Input: part model. Units: mm. Frame: model coordinates. Face numbers are marked on the shaded views. A direction names the side the tool comes from. Give positions to 0.01 mm unless a question says otherwise; leave off trailing zeros. Order: outer loops, then holes, each group sorted by start corner. A loop starts at its lowest first (then second) coordinate and runs counter-clockwise, first axis right, second up. Notation, with made-up numbers: (10.5, 46) - (55.5, 46) arc R19 cw to (55.5, 69) - close; hole circle Ø11 at (25.5, 89). An arc over 180 degrees is marked (long way). Answer in a Markdown table with one row per item. Add a question column.
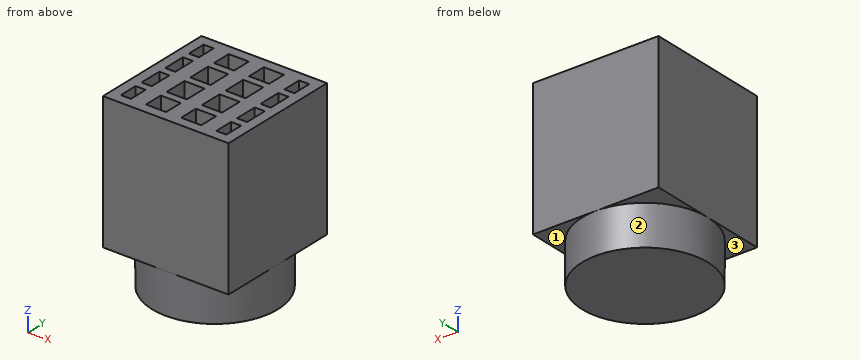
from build123d import *

# Parameters (mm, degrees)
SKETCH_8_W       = 25
SKETCH_8_H       = 25
SKETCH_8_W_2     = 4
SKETCH_8_H_2     = 21
SKETCH_8_W_3     = 2
EXTRUDE_7_DEPTH  = 25
SKETCH_9_W       = 25
SKETCH_9_H       = 25
EXTRUDE_8_DEPTH  = 2
SKETCH_14_W      = 25
SKETCH_14_H      = 1.5
EXTRUDE_11_DEPTH = 25
SKETCH_16_R      = 12.5
SKETCH_16_R_2    = 10
EXTRUDE_14_DEPTH = 6
SKETCH_17_R      = 12.5
EXTRUDE_15_DEPTH = 2


with BuildPart() as part:
    # 草图8 → 凸台-拉伸7 (new body)
    with BuildSketch(Plane.XY):
        Rectangle(SKETCH_8_W, SKETCH_8_H)
        with Locations((3.5, 0)):
            Rectangle(SKETCH_8_W_2, SKETCH_8_H_2, mode=Mode.SUBTRACT)
        with Locations((-3.5, 0)):
            Rectangle(SKETCH_8_W_2, SKETCH_8_H_2, mode=Mode.SUBTRACT)
        with Locations((-9.5, 0)):
            Rectangle(SKETCH_8_W_3, SKETCH_8_H_2, mode=Mode.SUBTRACT)
        with Locations((9.5, 0)):
            Rectangle(SKETCH_8_W_3, SKETCH_8_H_2, mode=Mode.SUBTRACT)
    extrude(amount=EXTRUDE_7_DEPTH)

    # 草图9 → 凸台-拉伸8 (add)
    with BuildSketch(Plane(origin=(0, 0, 0), x_dir=(-1, 0, 0), z_dir=(0, 0, -1))):
        Rectangle(SKETCH_9_W, SKETCH_9_H)
    extrude(amount=EXTRUDE_8_DEPTH)

    # 草图14 → 凸台-拉伸11 (add)
    with BuildSketch(Plane.XY.offset(25)):
        Rectangle(SKETCH_14_W, SKETCH_14_H)
        with Locations((0, 6)):
            Rectangle(SKETCH_14_W, SKETCH_14_H)
        with Locations((0, -6)):
            Rectangle(SKETCH_14_W, SKETCH_14_H)
    extrude(amount=-EXTRUDE_11_DEPTH)

    # 草图16 → 凸台-拉伸14 (add)
    with BuildSketch(Plane(origin=(0, 0, -2), x_dir=(-1, 0, 0), z_dir=(0, 0, -1))):
        Circle(SKETCH_16_R)
        Circle(SKETCH_16_R_2, mode=Mode.SUBTRACT)
    extrude(amount=EXTRUDE_14_DEPTH)

    # 草图17 → 凸台-拉伸15 (add)
    with BuildSketch(Plane(origin=(0, 0, -8), x_dir=(-1, 0, 0), z_dir=(0, 0, -1))):
        Circle(SKETCH_17_R)
    extrude(amount=EXTRUDE_15_DEPTH)


solid = part.part
Q1. Section A-A, the plane y = -6. Return loops of the section in (x, z), then the cut area to 3 significant figures.
Q2. Section B-B, the plane z = 15.5. State how many separate pieces and enclosed holes the cut face has, then the cut area to 3 significant figures.
Q3. Contact query for a flat-ended pin moving along its axis: P1, Ø1.2, axis at x = -2.5, y = -2.5, coming from the +Z side. Output: stop coordinate, or through.
Q4. Line query: probe 1 along X at (y, z) = (1.5, 19); probe 2 along Z at (x, y) = (-5, -2.25); probe 3 along Y at (x, z) = (0, -4.3). Output: solid intervals per line, ascending.
Q5. Section C-C, the plane x = 1. Return loops of the section in (y, z), then the cut area to 3 significant figures.
Q6. Section D-D, the plane x = -5. Return loops of the section in (y, z), then the cut area to 3 significant figures.
Q7. Access query for the marked faces 1, 2 and 3. Directions: +Z, -Z, +X, -X, +Y, -Y. A direction counts if a zero-diameter tool reaches every point of the face in a straight line with its end or side. Return the directions, or none.
Computed:
| question | item | result |
|---|---|---|
| 1 | outline | (-12.5, -2) - (-10.97, -2) - (-10.97, -10) - (10.97, -10) - (10.97, -2) - (12.5, -2) - (12.5, 25) - (-12.5, 25) - close; hole (-8, -8) - (8, -8) - (8, -2) - (-8, -2) - close |
| 1 | area | 754 mm^2 |
| 2 | separate pieces | 1 |
| 2 | enclosed holes | 16 |
| 2 | area | 427 mm^2 |
| 3 | P1 | stops at z = 0 |
| 4 | probe 1 | x = -12.5 to -10.5, -8.5 to -5.5, -1.5 to 1.5, 5.5 to 8.5, 10.5 to 12.5 |
| 4 | probe 2 | z = -10 to -8, -2 to 0 |
| 4 | probe 3 | y = -12.5 to -10, 10 to 12.5 |
| 5 | outline | (-12.5, -2) - (-12.46, -2) - (-12.46, -10) - (12.46, -10) - (12.46, -2) - (12.5, -2) - (12.5, 25) - (-12.5, 25) - close; hole (-9.95, -8) - (9.95, -8) - (9.95, -2) - (-9.95, -2) - close |
| 5 | area | 755 mm^2 |
| 6 | outline | (-12.5, -2) - (-11.46, -2) - (-11.46, -10) - (11.46, -10) - (11.46, -2) - (12.5, -2) - (12.5, 25) - (10.5, 25) - (10.5, 0) - (6.75, 0) - (6.75, 25) - (5.25, 25) - (5.25, 0) - (0.75, 0) - (0.75, 25) - (-0.75, 25) - (-0.75, 0) - (-5.25, 0) - (-5.25, 25) - (-6.75, 25) - (-6.75, 0) - (-10.5, 0) - (-10.5, 25) - (-12.5, 25) - close; hole (-8.66, -8) - (8.66, -8) - (8.66, -2) - (-8.66, -2) - close |
| 6 | area | 342 mm^2 |
| 7 | face 1 | -Z, +X, +Y |
| 7 | face 2 | -Z |
| 7 | face 3 | -Z, -X, -Y |
